from build123d import *

# Parameters (mm, degrees)
F1_DEPTH = 40
F2_R     = 2.5
F3_DEPTH = 100.001
F4_R     = 1.5
F5_DEPTH = 20


with BuildPart() as f1:
    # F0 (on Front) → F1 (new body)
    with BuildSketch(Plane.XZ):
        with BuildLine():
            Line((0, 150), (0, 0))
            Line((0, 0), (100, 0))
            add(Edge.make_bspline(
                [(0, 150), (33.333333, 100), (66.666667, 50), (100, 0)],
                knots=[0, 0, 0, 0, 180.277564, 180.277564, 180.277564, 180.277564], degree=3))
        make_face()
    extrude(amount=F1_DEPTH)

    # F2 (on face) → F3 (cut, through all)
    with BuildSketch(Plane(origin=(0, 0, 0), x_dir=(0, -1, 0), z_dir=(-1, 0, 0))):
        with Locations((20, 25)):
            Circle(F2_R)
    extrude(amount=-F3_DEPTH, mode=Mode.SUBTRACT)

    # F4 (on face) → F5 (cut)
    with BuildSketch(Plane(origin=(0, 0, 0), x_dir=(0, -1, 0), z_dir=(-1, 0, 0))):
        with Locations((20, 57)):
            Circle(F4_R)
        with Locations((20, 44)):
            Circle(F4_R)
    extrude(amount=-F5_DEPTH, mode=Mode.SUBTRACT)


solid = f1.part
CAD build for the part. Positions are in the model's coordinates, mm. A direction names the side the tool comes from. Give positions to 0.01 mm unless a question says otherwise; leave off trailing zeros. Answer as CSV lines item,"result".
Q1. Pull direction Z, two halves, no side cores. Call faces 3 (the face through (27, -40, 43)), 4 (the face through (9.86, -19.675, 42.536)), 5 (the face through (49, -20, 0)): released by +Z, released by -Z, zero draft, split by the parting line, or undercut.
Result set:
face 3,"zero draft"
face 4,"undercut"
face 5,"released by -Z"
Q2. Flat gauge pins, fed straight in: pin 1 Ø2.5 at (y, z) = (-20, 57) entering from +X; pin 2 Ø10 at (x, y) = (29.5, -6) entering from +Z; pin 3 Ø1.8 at (y, z) = (-20, 44) entering from -X. Where does each tip first touch, or does it go through?
Result set:
pin 1,"x = 62.83"
pin 2,"z = 113.25"
pin 3,"x = 20"
Q3. Drill centre lines: line 1 (Z direction, x = 12, y = -20); line 2 (Z direction, x = 4.75, y = -20) (3 decimals); line 3 (Z direction, x = 28.5, y = -20). Where is each one in solid material? Low to high. Write a range as from..to.
Result set:
line 1,"0..22.5, 27.5..42.5, 45.5..55.5, 58.5..132"
line 2,"0..22.5, 27.5..42.5, 45.5..55.5, 58.5..142.875"
line 3,"0..22.5, 27.5..107.25"
Q4. 3-axis set-ups, long thin cutter, end or side, ignore diameter. For faces 1 (the face through (41.91, -18.16, 26.69)), 2 (the face through (9.86, -18.89, 58.01)): which of +Z, -Z, +X, -X, +Y, -Y reach the whole face in a straight line?
Result set:
face 1,"+X, -X"
face 2,"-X"
